from build123d import *

# Parameters (mm, degrees)
F0_R     = 25.4
F0_R_2   = 3.2385
F0_R_3   = 8
F1_DEPTH = 4.7625
F2_W     = 50.561215
F2_H     = 14.34433
F3_DEPTH = 25.4
F5_DEPTH = 2.38125


with BuildPart() as f1:
    # F0 (on Front) → F1 (new body)
    with BuildSketch(Plane.XZ):
        Circle(F0_R)
        with Locations((0, -16.6624)):
            Circle(F0_R_2, mode=Mode.SUBTRACT)
        Circle(F0_R_3, mode=Mode.SUBTRACT)
        with Locations((-14.430062, 8.3312)):
            Circle(F0_R_2, mode=Mode.SUBTRACT)
        with Locations((14.430062, 8.3312)):
            Circle(F0_R_2, mode=Mode.SUBTRACT)
    extrude(amount=F1_DEPTH)

    # F2 (on face) → F3 (cut)
    with BuildSketch(Plane.XZ.offset(4.7625)):
        with Locations((0.75591, 26.222165)):
            Rectangle(F2_W, F2_H)
    extrude(amount=-F3_DEPTH, mode=Mode.SUBTRACT)

    # F4 (on face) → F5 (cut)
    with BuildSketch(Plane.XZ.offset(4.7625)):
        with BuildLine():
            ThreePointArc((-3.646079, -10.497322), (-9.623707, -5.55625), (-10.913987, 2.091064))
            ThreePointArc((-10.913987, 2.091064), (-11.409826, 3.527057), (-12.900289, 3.821078))
            ThreePointArc((-12.900289, 3.821078), (-16.190201, 3.905896), (-18.639619, 6.103863))
            ThreePointArc((-18.639619, 6.103863), (-20.156405, 6.905634), (-21.458089, 5.788007))
            ThreePointArc((-21.458089, 5.788007), (-19.247415, -11.1125), (-5.716484, -21.477254))
            ThreePointArc((-5.716484, -21.477254), (-4.097748, -20.908775), (-4.033709, -19.194315))
            ThreePointArc((-4.033709, -19.194315), (-4.712495, -15.974073), (-3.140994, -13.082517))
            ThreePointArc((-3.140994, -13.082517), (-2.650392, -11.644727), (-3.646079, -10.497322))
        make_face()
        with BuildLine():
            ThreePointArc((-7.267908, 8.406258), (0, 11.1125), (7.267908, 8.406258))
            ThreePointArc((7.267908, 8.406258), (8.759433, 8.11767), (9.759295, 9.261439))
            ThreePointArc((9.759295, 9.261439), (10.905182, 11.533797), (13.057597, 12.891655))
            ThreePointArc((13.057597, 12.891655), (14.126157, 14.572961), (12.618408, 15.875))
            Line((12.618408, 15.875), (-12.618408, 15.875))
            ThreePointArc((-12.618408, 15.875), (-14.126157, 14.572961), (-13.057597, 12.891655))
            ThreePointArc((-13.057597, 12.891655), (-10.905182, 11.533797), (-9.759295, 9.261439))
            ThreePointArc((-9.759295, 9.261439), (-8.759433, 8.11767), (-7.267908, 8.406258))
        make_face()
        with BuildLine():
            ThreePointArc((10.913987, 2.091064), (9.623707, -5.55625), (3.646079, -10.497322))
            ThreePointArc((3.646079, -10.497322), (2.650392, -11.644727), (3.140994, -13.082517))
            ThreePointArc((3.140994, -13.082517), (4.712495, -15.974073), (4.033709, -19.194315))
            ThreePointArc((4.033709, -19.194315), (4.097748, -20.908775), (5.716484, -21.477254))
            ThreePointArc((5.716484, -21.477254), (19.247415, -11.1125), (21.458089, 5.788007))
            ThreePointArc((21.458089, 5.788007), (20.156405, 6.905634), (18.639619, 6.103863))
            ThreePointArc((18.639619, 6.103863), (16.190201, 3.905896), (12.900289, 3.821078))
            ThreePointArc((12.900289, 3.821078), (11.409826, 3.527057), (10.913987, 2.091064))
        make_face()
    extrude(amount=-F5_DEPTH, mode=Mode.SUBTRACT)


solid = f1.part
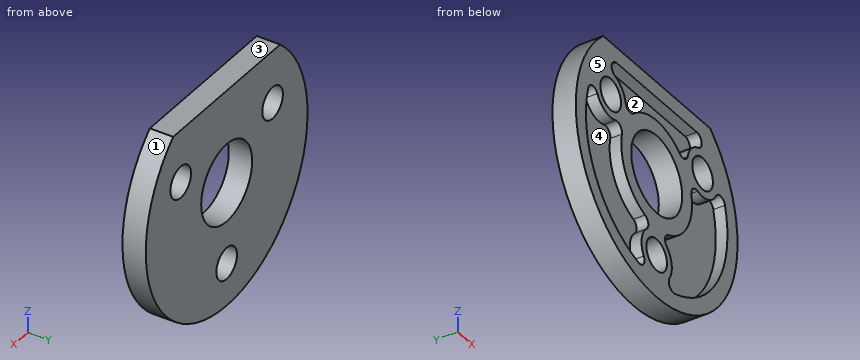
Source: CAD feature listing. Evaluate the final solid. Frame: model axes, mm. Face numbers are marked on the shaded views. A direction names the side the tool comes from. Coordinates: 2 decimals unless noted, no trailing zeros. Loops run counter-clockwise (first coordinate to the right, second up) from the corner with the lowest first, then second, coordinate; pieces in that order, holes last. Notation, with made-up numbers: (0.25, -38) -> (31.25, -38) arc R31 cw to (31.25, -3) -> close; hole circle Ø5 at (45, 41). An arc over 180 degrees is marked (long way). Answer in a Markdown table with one row per item. Add a question column.
Q1. Ray query, line 1 along Z through (x, y) = (0, -1.7); line 2 along X through (y, z) = (-2.95, -15); line 3 along Z through (x, y) = (-2.5, -2.85) (3 decimals). Return the intervals inside material, ascending.
Q2. Section B-B on x = 0. Give the number of separate pieces and of enclosed holes in the cut face, and give its area (3 significant figures).
Q3. Pull-direction query (X, two-part tool) for the marked faces 1, 2 and 3; classes: pulls with the +X half, pulls with the -X half, needs draft (parallel to the pull), parting line crosses it, or undercut.
Q4. Contact query for flat-ended pins moving along their axis: pin 1 Ø9.5 at (x, z) = (0, 0) entering from -Y; pin 2 Ø0.7 at (x, y) = (-3.5, -3) entering from -Z. Output: stop coordinate, or through.
Q5. Section A-A on z = 0. Return the cut outline in (x, y) (1 decimal).
Q6. Section D-D on y = -0.9. Return the cut outline in (x, z), and give its area (3 significant figures).
Q7. Reachability of the marked faces 4 and 5 from +Z, -Z, +X, -X, +Y, -Y: full face, straight path, thin tool, end or side. Return the list, or none.
Computed values:
| question | item | result |
|---|---|---|
| 1 | line 1 | z = -25.4 to -19.9, -13.42 to -8, 8 to 19.05 |
| 1 | line 2 | x = -20.5 to -16.4, -4.46 to -2.78, 2.78 to 4.46, 16.4 to 20.5 |
| 1 | line 3 | z = -25.277 to -18.721, -14.604 to -7.599, 7.599 to 10.828, 15.875 to 19.05 |
| 2 | separate pieces | 3 |
| 2 | enclosed holes | 0 |
| 2 | area | 93.3 mm^2 |
| 3 | face 1 | parting line crosses it |
| 3 | face 2 | undercut |
| 3 | face 3 | needs draft |
| 4 | pin 1 | passes through |
| 4 | pin 2 | stops at z = -25.2 |
| 5 | outline | (-25.4, -4.8) -> (-22.2, -4.8) -> (-22.2, -2.4) -> (-11.1, -2.4) -> (-11.1, -4.8) -> (-8, -4.8) -> (-8, 0) -> (-25.4, 0) -> close; (8, -4.8) -> (11.1, -4.8) -> (11.1, -2.4) -> (22.2, -2.4) -> (22.2, -4.8) -> (25.4, -4.8) -> (25.4, 0) -> (8, 0) -> close |
| 6 | outline | (-16.8, 19.05) arc R25.4 ccw (long way) to (16.8, 19.05) -> close; hole circle Ø6.48 at (-14.43, 8.33); hole circle Ø16 at (0, 0); hole circle Ø6.48 at (0, -16.66); hole circle Ø6.48 at (14.43, 8.33) |
| 6 | area | 1,580 mm^2 |
| 7 | face 4 | -Y |
| 7 | face 5 | +Z, -Z, +X, -X, -Y |
